Autodesk Fusion 360 part; units mm, degrees
sketch "Sketch1" plane through (0, 0, 0) normal (0, 1, 0) x (1, 0, 0)
  line L0 (3, 1.7321) -> (0, 3.4641)
  line L1 (0, 3.4641) -> (-3, 1.7321)
  line L2 (-3, 1.7321) -> (-3, -1.7321)
  line L3 (-3, -1.7321) -> (0, -3.4641)
  line L4 (0, -3.4641) -> (3, -1.7321)
  line L5 (3, -1.7321) -> (3, 1.7321)
  dimension "d1" = 3
extrude "Extrude1" add sketch "Sketch1" along normal blind 40
sketch "Sketch4" plane through (0, 40, 0) normal (0, 1, 0) x (-1, 0, 0)
  line L0 (0, 3.4641) -> (-3, 1.7321)
  line L1 (-3, 1.7321) -> (-3, -1.7321)
  line L2 (-3, -1.7321) -> (0, -3.4641)
  line L3 (0, -3.4641) -> (3, -1.7321)
  line L4 (3, -1.7321) -> (3, 1.7321)
  line L5 (3, 1.7321) -> (0, 3.4641)
  circle A0 centre (0, 0) radius 1.5
  line L6 (-3, 1.7321) -> (-3, -1.7321)
  line L7 (-3, -1.7321) -> (0, -3.4641)
  line L8 (0, -3.4641) -> (3, -1.7321)
  line L9 (3, -1.7321) -> (3, 1.7321)
  line L10 (3, 1.7321) -> (0, 3.4641)
  line L11 (0, 3.4641) -> (-3, 1.7321)
  dimension "d8" = 3
extrude "Extrude4" cut sketch "Sketch4" against normal blind 6 contours A0
thread "Thread1"
sketch "Sketch5" plane through (0, 0, 0) normal (0, -1, 0) x (1, 0, 0)
  line L0 (3, -1.7321) -> (3, 1.7321)
  line L1 (3, 1.7321) -> (0, 3.4641)
  line L2 (0, 3.4641) -> (-3, 1.7321)
  line L3 (-3, 1.7321) -> (-3, -1.7321)
  line L4 (-3, -1.7321) -> (0, -3.4641)
  line L5 (0, -3.4641) -> (3, -1.7321)
  circle A0 centre (0, 0) radius 1.5
  dimension "d11" = 3
extrude "Extrude5" cut sketch "Sketch5" against normal blind 6 contours A0
thread "Thread2"
Verification items for the finished model (mm, model axes). A direction names the side the tool comes from. Coordinates: 2 decimals unless noted, no trailing zeros. Write each loop counter-clockwise with the first axis right and the second up, starting at its lowest first coordinate (ties: lowest second). Pieces come first, ordered by that corner, then holes. Notation, with made-up numbers: M 2,76 L 41,76 A20 ccw 41,94 Z; hole C 28.25,-27 d6. An arc over 180 degrees is marked long. One line per item, written item: value.
Item 1: Section check B-B, the plane z = 0. Record the boundary of the cut face in (x, y).
Check sheet entries:
outline: M -3,0 L -1.5,0 L -1.5,6 L 1.5,6 L 1.5,0 L 3,0 L 3,40 L 1.5,40 L 1.5,34 L -1.5,34 L -1.5,40 L -3,40 Z
Item 2: Access from +Z, -Z, +X, -X, +Y, -Y to the whole of each face (thin tool, end or side, straight path). Record for faces 1 (the flat face through (0, 6, 0)), 2 (the flat face through (1.5, 19.7, 2.6)), 3 (the cylindrical face through (1.5, 37.04, 0.07)).
Check sheet entries:
face 1: -Y
face 2: +Z, +X, +Y, -Y
face 3: +Y
Item 3: Gauge pin test, flat ends, axial feed: pin 1 Ø2.5 at (x, z) = (0, 0) entering from +Y; pin 2 Ø0.9 at (x, z) = (0, 0.5) entering from -Y. Record the tip position at first contact, or that the pin passes through.
Check sheet entries:
pin 1: stops at y = 34
pin 2: stops at y = 6
Item 4: Mould release check, pull along Z, two halves, no side actions. Record for faces 4 (the cylindrical face through (-1.5, 2.96, 0.07)), 5 (the flat face through (1.5, 19.7, -2.6)), 6 (the flat face through (-1.5, 19.7, 2.6)): pulls with the +Z half, pulls with the -Z half, needs draft (parallel to the pull), parting line crosses it, or undercut.
Check sheet entries:
face 4: undercut
face 5: pulls with the -Z half
face 6: pulls with the +Z half
Item 5: Section check A-A, the plane y = 5. Record the boundary of the cut face in (x, z), plus the area to 3 significant figures.
Check sheet entries:
outline: M -3,-1.73 L 0,-3.46 L 3,-1.73 L 3,1.73 L 0,3.46 L -3,1.73 Z; hole C 0,0 d3
area: 24.1 mm^2
Item 6: Scan lines: line 1 along Z through (x, y) = (0.8, 31); line 2 along Z through (x, y) = (0.85, 36); line 3 along Y through (x, z) = (-1.25, -0.5). Record each from-to range of solid material in increasing order.
Check sheet entries:
line 1: z = -3 to 3
line 2: z = -2.97 to -1.24, 1.24 to 2.97
line 3: y = 6 to 34
Item 7: Section check D-D, the plane x = -2.2. Record the boundary of the cut face in (y, z), plus the area to 3 significant figures.
Check sheet entries:
outline: M 0,-2.19 L 40,-2.19 L 40,2.19 L 0,2.19 Z
area: 176 mm^2
Item 8: Section check C-C, the plane x = -0.4. Record the boundary of the cut face in (y, z), plus the area to 3 significant figures.
Check sheet entries:
outline: M 0,-3.23 L 40,-3.23 L 40,-1.45 L 34,-1.45 L 34,1.45 L 40,1.45 L 40,3.23 L 0,3.23 L 0,1.45 L 6,1.45 L 6,-1.45 L 0,-1.45 Z
area: 224 mm^2
